Here's the drawing with two shaded views (mm, measured from the low corner). I have some questions. A direction names the side the tool comes from. Give positions to 0.01 mm unless a question says otherwise; leave off trailing zeros. Write each loop counter-clockwise with the first axis right and the second up, starting at its lowest first coordinate (ties: lowest second). Pieces come first, ordered by that corner, then holes. Notation, with made-up numbers: (37, 70.25) - (67, 70.25) arc R31 ccw to (67, 102.25) - close; hole circle Ø3 at (11, 66). An arc over 180 degrees is marked (long way). Write item = value, one per line.
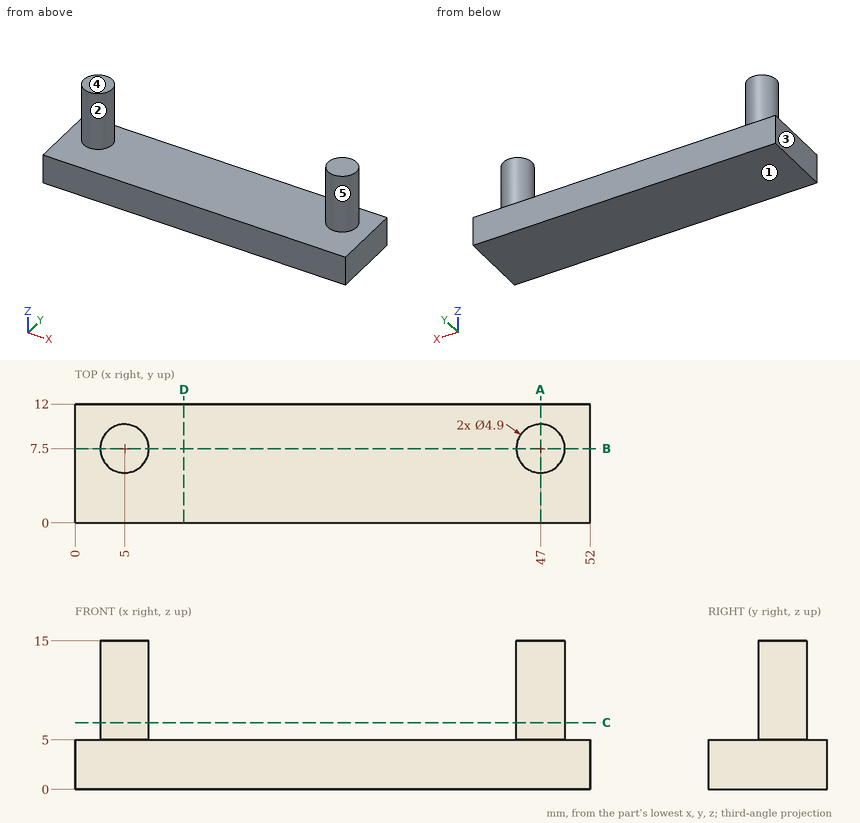
1. Which directions (+Z, -Z, +X, -X, +Y, -Y) give clear straight access to the entire face, cutting with the end or side of a thin tool? Please do the marked faces 4 and 5.
Filled sheet:
face_4 = +Z, +X, -X, +Y, -Y
face_5 = +Z
2. If we section it at A-A, the plane x = 47: Please give me the cut outline in (y, z).
Filled sheet:
outline = (0, 0) - (12, 0) - (12, 5) - (9.95, 5) - (9.95, 15) - (5.05, 15) - (5.05, 5) - (0, 5) - close
3. If we section it at B-B, the plane y = 7.5: Please give me the cut outline in (x, z), and give its area (3 significant figures).
Filled sheet:
outline = (0, 0) - (52, 0) - (52, 5) - (49.45, 5) - (49.45, 15) - (44.55, 15) - (44.55, 5) - (7.45, 5) - (7.45, 15) - (2.55, 15) - (2.55, 5) - (0, 5) - close
area = 358 mm2
4. Thinking about a two-plate mould opening in X: for the marked faces 1, 2 and 3, which applies, pulls with the +X half, pulls with the -X half, needs draft (parallel to the pull), parting line crosses it, or undercut?
Filled sheet:
face_1 = needs draft
face_2 = undercut
face_3 = pulls with the -X half
5. If we section it at C-C, the plane z = 6.75: Please give me the cut outline in (x, y).
Filled sheet:
outline = circle Ø4.9 at (5, 7.5); circle Ø4.9 at (47, 7.5)
6. I need wall thicknesses on line 1 (X direction, y = 8.5, z = 7.75); line 2 (Z direction, x = 4, y = 2.25); line 3 (Y direction, x = 5, z = 5.25). Which ranges of each line are inside material? Lowest first, please.
Filled sheet:
line_1 = 2.76 to 7.24, 44.76 to 49.24
line_2 = 0 to 5
line_3 = 5.05 to 9.95
7. If we section it at D-D, the plane x = 11: Please give me the cut outline in (y, z).
Filled sheet:
outline = (0, 0) - (12, 0) - (12, 5) - (0, 5) - close
8. For pin 1 (1.5 mm diameter, centred on x = 30, y = 10.5, fed in from -Z); pin 2 (5 mm diameter, centred on x = 37, y = 8, fed in from +Z); pin 3 (4 mm diameter, centred on x = 32, z = 7.5, fed in from +Y), each with a flat end and sliding along its axis, tell me the tip position at first contact or that it passes through.
Filled sheet:
pin_1 = 0
pin_2 = 5
pin_3 = through
